Read the model definition and answer for the solid it produces. Units are mm, in the model's axes. Face numbers are marked on the shaded views. A direction names the side the tool comes from. Round coordinates to 2 decimals unless told otherwise and drop trailing zeros. Loops run counter-clockwise (first coordinate to the right, second up) from the corner with the lowest first, then second, coordinate; pieces in that order, holes last. Notation, with made-up numbers: (74, -28) - (84, -28) arc R32 cw to (84, -1) - close; hole circle Ø2 at (-20.5, 5.25). An arc over 180 degrees is marked (long way). Use one line per item in the form item = value. Start each with the question number.
```python
from build123d import *

# Parameters (mm, degrees)
BOSS_EXTRUDE1_DEPTH     = 18
SKETCH3_W               = 33
SKETCH3_H               = 10
CUT_EXTRUDE1_DEPTH      = 143.562267098
CUT_EXTRUDE2_DEPTH      = 143.562267098
CUT_EXTRUDE3_DEPTH      = 143.562267098
CUT_EXTRUDE4_DEPTH      = 143.562267098
BOSS_EXTRUDE2_DEPTH     = 18
BOSS_EXTRUDE3_DEPTH     = 18
LPATTERN1_COUNT         = 30
LPATTERN1_PITCH         = 3
CUT_EXTRUDE5_DEPTH      = 146.668613805
CUT_EXTRUDE6_DEPTH      = 146.668613805
CUT_EXTRUDE7_DEPTH      = 146.668613805
CUT_EXTRUDE8_DEPTH      = 146.668613805
CUT_EXTRUDE9_DEPTH      = 4.5
CUT_EXTRUDE9_DEPTH_BACK = 4.5
FILLET1_R               = 5
F_6_0_MM_DOWEL_HOLES1_D = 6.2


with BuildPart() as part:
    # Sketch2 → Boss-Extrude1 (new body)
    with BuildSketch(Plane.XY):
        with BuildLine():
            Line((-20, 0), (20, 0))
            Line((20, 0), (20, 140))
            ThreePointArc((20, 140), (-9.083269132, 116.055512755), (-20, 80))
            Line((-20, 80), (-20, 0))
        make_face()
    extrude(amount=BOSS_EXTRUDE1_DEPTH)

    # Sketch3 → Cut-Extrude1 (cut, through all)
    with BuildSketch(Plane.XY.offset(18)):
        with Locations((0.5, 28)):
            Rectangle(SKETCH3_W, SKETCH3_H)
    extrude(amount=-CUT_EXTRUDE1_DEPTH, mode=Mode.SUBTRACT)

    # Sketch4 → Cut-Extrude2 (cut, through all)
    with BuildSketch(Plane.XY.offset(18)):
        Polygon((-16, 36), (17, 36), (17, 46), (-16, 51.818790363), align=None)
    extrude(amount=-CUT_EXTRUDE2_DEPTH, mode=Mode.SUBTRACT)

    # Sketch5 → Cut-Extrude3 (cut, through all)
    with BuildSketch(Plane.XY.offset(18)):
        Polygon((-16, 54.865070199), (17, 49.046279836), (17, 59.046279836), (-16, 71.057297566), align=None)
    extrude(amount=-CUT_EXTRUDE3_DEPTH, mode=Mode.SUBTRACT)

    # Sketch6 → Cut-Extrude4 (cut, through all)
    with BuildSketch(Plane.XY.offset(18)):
        with BuildLine():
            Line((-16, 74.249830884), (17, 62.238813153))
            Line((17, 62.238813153), (17, 72.238813153))
            Line((17, 72.238813153), (-15.046889298, 90.741093316))
            ThreePointArc((-15.046889298, 90.741093316), (-15.761255119, 85.391648765), (-16, 80))
            Line((-16, 80), (-16, 74.249830884))
        make_face()
    extrude(amount=-CUT_EXTRUDE4_DEPTH, mode=Mode.SUBTRACT)

    # Sketch13 → Boss-Extrude2 (add)
    with BuildSketch(Plane.XY.offset(18)):
        with BuildLine():
            Line((27.463865989, 141.919276749), (27.463865989, 139.919276749))
            ThreePointArc((27.463865989, 139.919276749), (21.883638711, 121.290161062), (20, 101.934676234))
            Line((20, 101.934676234), (20, 140))
            ThreePointArc((20, 140), (23.663152719, 141.227117654), (27.463865989, 141.919276749))
        make_face()
    extrude(amount=-BOSS_EXTRUDE2_DEPTH)

    # Sketch15 → Boss-Extrude3 (add)
    with BuildSketch(Plane.XY.offset(18)):
        Polygon((20, 101.934676234), (22.598076211, 100.434676234), (20, 98.934676234), align=None)
    boss_extrude3 = extrude(amount=-BOSS_EXTRUDE3_DEPTH)

    # LPattern1: Boss-Extrude3 ×30
    with Locations(*[(0, -i * LPATTERN1_PITCH, 0) for i in range(1, LPATTERN1_COUNT)]):
        add(boss_extrude3)

    # Sketch17 → Cut-Extrude5 (cut, through all)
    with BuildSketch(Plane.XY.offset(18)):
        with BuildLine():
            Line((-14.409820926, 93.837383335), (17, 75.702914768))
            Line((17, 75.702914768), (17, 85.702914768))
            Line((17, 85.702914768), (-9.308172311, 107.778092451))
            ThreePointArc((-9.308172311, 107.778092451), (-12.284651864, 100.963507838), (-14.409820926, 93.837383335))
        make_face()
    extrude(amount=-CUT_EXTRUDE5_DEPTH, mode=Mode.SUBTRACT)

    # Sketch18 → Cut-Extrude6 (cut, through all)
    with BuildSketch(Plane.XY.offset(18)):
        with BuildLine():
            Line((-7.846238812, 110.46760646), (17, 89.619136636))
            Line((17, 89.619136636), (17, 99.619136636))
            Line((17, 99.619136636), (-0.566824758, 120.554463152))
            ThreePointArc((-0.566824758, 120.554463152), (-4.464319866, 115.697073553), (-7.846238812, 110.46760646))
        make_face()
    extrude(amount=-CUT_EXTRUDE6_DEPTH, mode=Mode.SUBTRACT)

    # Sketch19 → Cut-Extrude7 (cut, through all)
    with BuildSketch(Plane.XY.offset(18)):
        with BuildLine():
            Line((1.497556464, 122.761400894), (17, 104.286308117))
            Line((17, 104.286308117), (17, 114.286308117))
            Line((17, 114.286308117), (8.554035532, 128.915147695))
            ThreePointArc((8.554035532, 128.915147695), (4.907555132, 125.973860666), (1.497556464, 122.761400894))
        make_face()
    extrude(amount=-CUT_EXTRUDE7_DEPTH, mode=Mode.SUBTRACT)

    # Sketch21 → Cut-Extrude8 (cut, through all)
    with BuildSketch(Plane.XY.offset(18)):
        with BuildLine():
            Line((11.013641865, 130.654984559), (17, 120.286308117))
            Line((17, 120.286308117), (17, 134.194095619))
            ThreePointArc((17, 134.194095619), (13.956345649, 132.509918344), (11.013641865, 130.654984559))
        make_face()
    extrude(amount=-CUT_EXTRUDE8_DEPTH, mode=Mode.SUBTRACT)

    # Sketch25 → Cut-Extrude9 (cut, two sides: drawn at the far end of the back side and taken through both)
    with BuildSketch(Plane(origin=(0, 0, 9), x_dir=(-1, 0, 0), z_dir=(0, 0, -1)).offset(-CUT_EXTRUDE9_DEPTH_BACK)):
        with BuildLine():
            Line((-20, 0), (-20, 7))
            Line((-20, 7), (-17, 7))
            ThreePointArc((-17, 7), (-14.171572875, 5.828427125), (-13, 3))
            Line((-13, 3), (-13, 0))
            Line((-13, 0), (-20, 0))
        make_face()
    extrude(amount=CUT_EXTRUDE9_DEPTH + CUT_EXTRUDE9_DEPTH_BACK, mode=Mode.SUBTRACT)

    # Fillet1
    fillet1_edges = [part.edges().sort_by_distance(p)[0] for p in [
        (20, 0, 2.25),
        (20, 0, 15.75),
        (-20, 0, 9),
    ]]
    fillet(fillet1_edges, radius=FILLET1_R)

    # Ø6.0 mm Dowel Holes1 (through all)
    with Locations(Plane.XY.offset(18)):
        with Locations((-15, 5)):
            f_6_0_mm_dowel_holes1 = Hole(F_6_0_MM_DOWEL_HOLES1_D / 2)

    # Mirror1: Ø6.0 mm Dowel Holes1 across plane
    add(f_6_0_mm_dowel_holes1.mirror(Plane(origin=(0, 0, 0), x_dir=(0, 0, 1), z_dir=(1, 0, 0))), mode=Mode.SUBTRACT)


solid = part.part
```
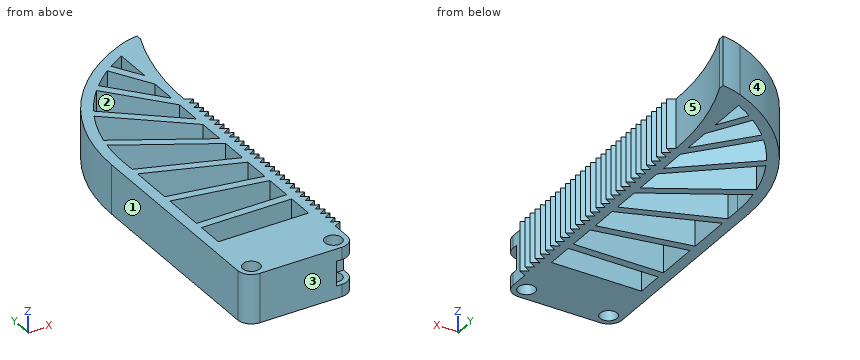
1) Flat-ended cylindrical pins translate along their axes: pin 1 (1.5 mm diameter, centred on x = 10, z = 13, fed in from +Y); pin 2 (1.5 mm diameter, centred on x = 19.5, z = 12, fed in from -Y); pin 3 (3 mm diameter, centred on y = 77.5, z = 11, fed in from +X). Find the tip coordinate at first contact, or state that the pin passes through.
2) A cutting plane is placed at A-A on y = 112. Write down the section's boundary in (x, z).
3) For the marked faces 1 and 2, determine the directions among +Z, -Z, +X, -X, +Y, -Y from which every point of the face is accessible in a straight line to the end or side of a thin tool.
4) A cutting plane is placed at B-B on z = 9.5. Count the separate pieces of the cut face and the enclosed holes in it, plus the area to 3 significant figures.
5) Determine the mould class of the marked faces 3, 4 and 5 for opening direction Y: +Y half, -Y half, draft (parallel to the pull), parting line (faces both ways), or undercut.
6) Straight lines are drawn through the part: line 1 (X direction, y = 86, z = 7.25); line 2 (X direction, y = 112, z = 10.75); line 3 (X direction, y = 56, z = 8.75). For each, find the intervals that lie inside material, in ascending order. Write a range as from..to.
Checks:
q1.pin_1 = 135.24
q1.pin_2 = 7
q1.pin_3 = 22.6
q2.outline = (-11.58, 0) - (-6.93, 0) - (-6.93, 18) - (-11.58, 18) - close; (6.61, 0) - (10.53, 0) - (10.53, 18) - (6.61, 18) - close; (17, 0) - (20.51, 0) - (20.51, 18) - (17, 18) - close
q3.face_1 = +Z, -Z, -X, +Y, -Y
q3.face_2 = +Z, -Z
q4.separate_pieces = 1
q4.enclosed_holes = 9
q4.area = 2,540 mm²
q5.face_3 = -Y half
q5.face_4 = +Y half
q5.face_5 = undercut
q6.line_1 = -19.72..-15.7, -6.84..-0.84, 16.65..21.62
q6.line_2 = -11.58..-6.93, 6.61..10.53, 17..20.51
q6.line_3 = -20..-16, 17..21.62
